Could you check a few things on this model? Use its own coordinates, in mm. Face numbers are marked on the shaded views. A direction names the side the tool comes from. Coordinates: 2 decimals unless noted, no trailing zeros. Loops run counter-clockwise (first coordinate to the right, second up) from the corner with the lowest first, then second, coordinate; pieces in that order, holes last. Notation, with made-up numbers: M 55,85.25 L 63,85.25 A19 cw 63,102.25 Z; hole C 18.25,27.5 d3. An arc over 180 degrees is marked long. Write each question's results on one line, items separated by ' | '.
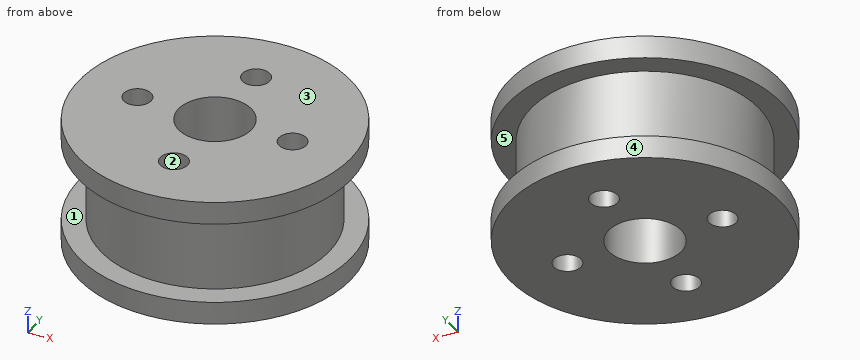
```python
from build123d import *

# Parameters (mm, degrees)
SKETCH1_R           = 14.9
SKETCH1_R_2         = 4
BOSS_EXTRUDE1_DEPTH = 14
SKETCH2_R           = 14.9
SKETCH2_R_2         = 12.5
CUT_EXTRUDE1_DEPTH  = 9
SKETCH3_R           = 1.5
CUT_EXTRUDE2_DEPTH  = 26.298616563


with BuildPart() as part:
    # Sketch1 → Boss-Extrude1 (new body)
    with BuildSketch(Plane.XY):
        Circle(SKETCH1_R)
        Circle(SKETCH1_R_2, mode=Mode.SUBTRACT)
    extrude(amount=BOSS_EXTRUDE1_DEPTH)

    # Sketch2 → Cut-Extrude1 (cut)
    with BuildSketch(Plane(origin=(0, 0, 2.5), x_dir=(-1, 0, 0), z_dir=(0, 0, -1))):
        Circle(SKETCH2_R)
        Circle(SKETCH2_R_2, mode=Mode.SUBTRACT)
    extrude(amount=-CUT_EXTRUDE1_DEPTH, mode=Mode.SUBTRACT)

    # Sketch3 → Cut-Extrude2 (cut, through all)
    with BuildSketch(Plane(origin=(0, 0, 0), x_dir=(-1, 0, 0), z_dir=(0, 0, -1))):
        with Locations((0, 8.5)):
            Circle(SKETCH3_R)
        with Locations((8.5, 0)):
            Circle(SKETCH3_R)
        with Locations((0, -8.5)):
            Circle(SKETCH3_R)
        with Locations((-8.5, 0)):
            Circle(SKETCH3_R)
    extrude(amount=-CUT_EXTRUDE2_DEPTH, mode=Mode.SUBTRACT)


solid = part.part
```
(1) If we mould it in two halves opening along Z, with no side actions, what happens to the marked faces 3, 4 and 5? For each: released by +Z, released by -Z, zero draft, split by the parting line, or undercut.
Reported:
face 3: released by +Z | face 4: zero draft | face 5: undercut
(2) Will these pins go through, and if not, where does the flat tip stop? P1, Ø2.5, axis at x = -8.5, y = 0, coming from the +Z side; P2, Ø2, axis at y = 9.5, z = 9, coming from the +X side; P3, Ø4, axis at y = -5, z = 7.5, coming from the -X side; P4, Ø5, axis at x = -6, z = 10.5, coming from the +Y side.
Reported:
P1: passes through | P2: stops at x = 9.17 | P3: stops at x = -12.13 | P4: stops at y = 14.43
(3) Imagine slicing it at C-C, the plane x = -8.5. List the corners of the cut face in (y, z) for me.
Reported:
outline: M -12.24,0 L -1.5,0 L -1.5,14 L -12.24,14 L -12.24,11.5 L -9.17,11.5 L -9.17,2.5 L -12.24,2.5 Z; M 1.5,0 L 12.24,0 L 12.24,2.5 L 9.17,2.5 L 9.17,11.5 L 12.24,11.5 L 12.24,14 L 1.5,14 Z
(4) Which directions (+Z, -Z, +X, -X, +Y, -Y) give clear straight access to the entire face, cutting with the end or side of a thin tool? Please do the marked faces 1 and 2.
Reported:
face 1: none | face 2: +Z, -Z
(5) Please list where these lines run through material, in increasing order: probe 1 along Y at (x, z) = (0, 9.75); probe 2 along Z at (x, y) = (-0.5, -13); probe 3 along X at (y, z) = (-2.5, 5.5). Write a range as from..to.
Reported:
probe 1: y = -12.5..-10, -7..-4, 4..7, 10..12.5 | probe 2: z = 0..2.5, 11.5..14 | probe 3: x = -12.25..-3.12, 3.12..12.25
(6) Imagine slicing it at A-A, the plane y = 0. List the corners of the cut face in (x, z) for me.
Reported:
outline: M -14.9,0 L -10,0 L -10,14 L -14.9,14 L -14.9,11.5 L -12.5,11.5 L -12.5,2.5 L -14.9,2.5 Z; M -7,0 L -4,0 L -4,14 L -7,14 Z; M 4,0 L 7,0 L 7,14 L 4,14 Z; M 10,0 L 14.9,0 L 14.9,2.5 L 12.5,2.5 L 12.5,11.5 L 14.9,11.5 L 14.9,14 L 10,14 Z
(7) Imagine slicing it at B-B, the plane z = 2. List the corners of the cut face in (x, y) for me.
Reported:
outline: C 0,0 d29.8; hole C -8.5,0 d3; hole C 0,0 d8; hole C 0,-8.5 d3; hole C 0,8.5 d3; hole C 8.5,0 d3
